Here's the drawing with two shaded views (mm, measured from the low corner). I have some questions. A direction names the side the tool comes from. Coordinates: 2 decimals unless noted, no trailing zeros. Loops run counter-clockwise (first coordinate to the right, second up) from the corner with the lowest first, then second, coordinate; pieces in that order, holes last.
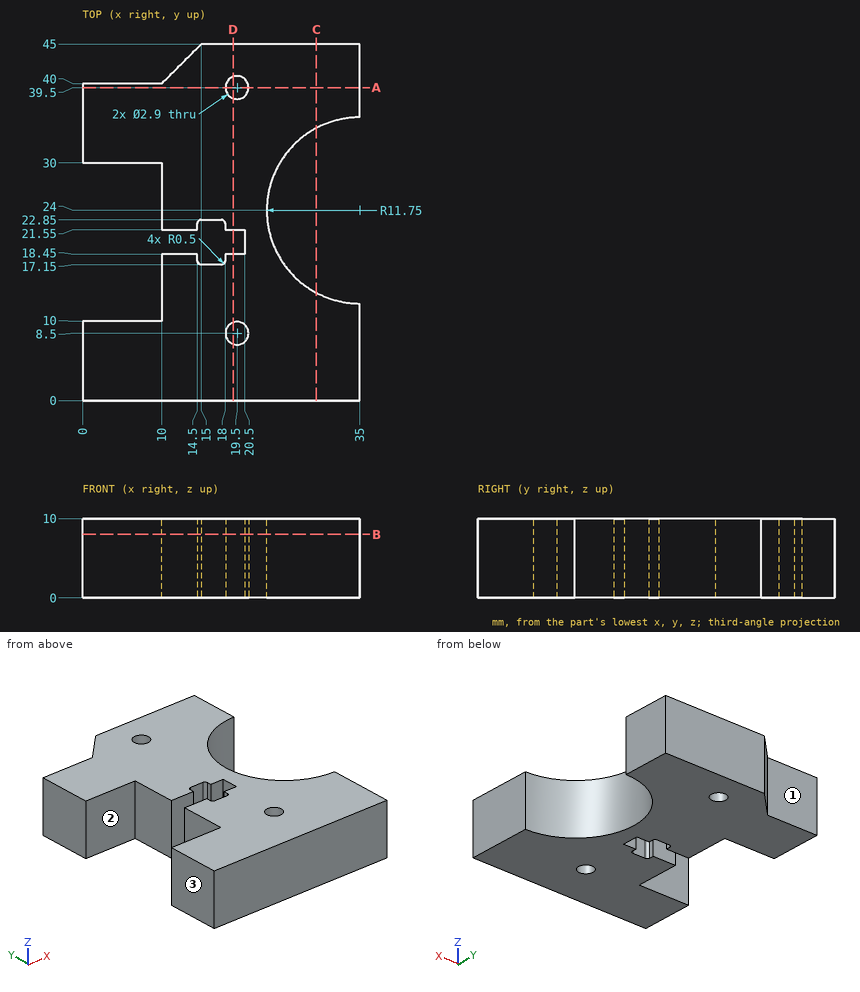
Q1. Suppose I cut it at A-A on y = 39.5. Write out the boundary of the cut face in (x, z).
Q2. Suppose I cut it at B-B on z = 8. State how many separate pieces and enclosed holes the cut face has, and give its area (3 significant figures).
Q3. For the marked faces 1, 2 and 3, which set-ups out of +Z, -Z, +X, -X, +Y, -Y let a thin tool reach every point of the face, with its end or its side?
Q4. Will these pins go through, and if not, where does the flat tip stop? P1, Ø1.5, axis at y = 22, z = 7.5, coming from the -X side; P2, Ø0.6, axis at y = 22, z = 6, coming from the +X side; P3, Ø3, axis at y = 31.5, z = 6, coming from the +X side.
Q5. Suppose I cut it at C-C on x = 29.5. Write out the boundary of the cut face in (y, z).
Q6. Please list where these lines run through material, in increasing order: probe 1 along Y at (x, z) = (19.5, 5.25); probe 2 along Y at (x, z) = (9, 9.75); probe 3 along X at (y, z) = (8.5, 6).
Q7. Suppose I cut it at D-D on x = 19. Write out the boundary of the cut face in (y, z).
Check values:
1. outline: (0, 0) - (18.05, 0) - (18.05, 10) - (0, 10) - close; (20.95, 0) - (35, 0) - (35, 10) - (20.95, 10) - close
2. separate pieces: 1
2. enclosed holes: 2
2. area: 1,040 mm2
3. face 1: +Z, -Z, -X, +Y
3. face 2: +Z, -Z, -X
3. face 3: +Z, -Z, -X, +Y, -Y
4. P1: stops at x = 10
4. P2: stops at x = 23.48
4. P3: stops at x = 27.45
5. outline: (0, 0) - (13.62, 0) - (13.62, 10) - (0, 10) - close; (34.38, 0) - (45, 0) - (45, 10) - (34.38, 10) - close
6. probe 1: y = 0 to 7.05, 9.95 to 18.45, 21.55 to 38.05, 40.95 to 45
6. probe 2: y = 0 to 10, 30 to 40
6. probe 3: x = 0 to 18.05, 20.95 to 35
7. outline: (0, 0) - (7.14, 0) - (7.14, 10) - (0, 10) - close; (9.86, 0) - (18.45, 0) - (18.45, 10) - (9.86, 10) - close; (21.55, 0) - (38.14, 0) - (38.14, 10) - (21.55, 10) - close; (40.86, 0) - (45, 0) - (45, 10) - (40.86, 10) - close
